Could you check a few things on this model? Use its own coordinates, in mm. Give positions to 0.01 mm unless a question says otherwise; leave off trailing zeros. Order: outer loops, then holes, each group sorted by start corner. A loop starts at its lowest first (then second) coordinate and runs counter-clockwise, first axis right, second up. Notation, with made-up numbers: (30.5, 29) - (71.5, 29) arc R19 cw to (71.5, 50) - close; hole circle Ø5 at (23, 59.5). An arc over 180 degrees is marked (long way). One line per question, with ' | ' between items. Start each with the question number.
1. For P1, Ø2, axis at y = -21, z = 1.5, coming from the -X side; P2, Ø1.6, axis at x = -21, z = 1.5, coming from the -Y side; P3, Ø3, axis at x = 10, y = 0, coming from the -Z side; P4, Ø4, axis at y = -3, z = 6, coming from the +X side, each with a flat end and sliding along its axis, tell me the tip position at first contact or that it passes through.
2. If we mould it in two halves opening along X, with no side actions, what happens to faces 1 (the flat face through (-21, 0.75, 1)), 2 (the flat face through (0, -5, 10)), 3 (the cylindrical face through (-0.228, -8.265, 6.056))? For each: released by +X, released by -X, zero draft, split by the parting line, or undercut.
3. Imagine slicing it at C-C (z = 3.5). Please give me the cut outline in (x, y).
4. I need wall thicknesses on probe 1 along Y at (x, z) = (0, 6); probe 2 along Y at (x, z) = (19, 1.25); probe 3 along Z at (x, y) = (18.5, 3). Which ranges of each line are inside material? Lowest first, please. Write a range as from..to.
5. Imagine slicing it at A-A (y = 0). Please give me the cut outline in (x, z), and give its area (3 significant figures).
```python
from build123d import *

# Parameters (mm, degrees)
SKETCH1_R           = 25
BOSS_EXTRUDE1_DEPTH = 10
SKETCH2_R           = 23
CUT_EXTRUDE1_DEPTH  = 2
SKETCH3_R           = 4
SKETCH3_R_2         = 1.75
CUT_EXTRUDE2_DEPTH  = 37.742346142
BOSS_EXTRUDE2_START = 2
BOSS_EXTRUDE2_DEPTH = 2
CIRPATTERN1_COUNT   = 20


with BuildPart() as part:
    # Sketch1 → Boss-Extrude1 (new body)
    with BuildSketch(Plane.XY):
        Circle(SKETCH1_R)
    extrude(amount=BOSS_EXTRUDE1_DEPTH)

    # Sketch2 → Cut-Extrude1 (cut)
    with BuildSketch(Plane(origin=(0, 0, 0), x_dir=(-1, 0, 0), z_dir=(0, 0, -1))):
        Circle(SKETCH2_R)
    extrude(amount=-CUT_EXTRUDE1_DEPTH, mode=Mode.SUBTRACT)

    # Sketch3 → Cut-Extrude2 (cut, through all)
    with BuildSketch(Plane.XY.offset(10)):
        Circle(SKETCH3_R)
        with Locations((10, 0)):
            Circle(SKETCH3_R_2)
        with Locations((0, -10)):
            Circle(SKETCH3_R_2)
        with Locations((-10, 0)):
            Circle(SKETCH3_R_2)
        with Locations((0, 10)):
            Circle(SKETCH3_R_2)
    extrude(amount=-CUT_EXTRUDE2_DEPTH, mode=Mode.SUBTRACT)

    # Sketch4 → Boss-Extrude2 (add)
    with BuildSketch(Plane(origin=(0, 0, 2), x_dir=(-1, 0, 0), z_dir=(0, 0, -1)).offset(BOSS_EXTRUDE2_START)):
        with BuildLine():
            Line((-0.75, 22.987768487), (-0.75, 18.464528853))
            Line((-0.75, 18.464528853), (0.75, 18.464528853))
            Line((0.75, 18.464528853), (0.75, 22.987768487))
            ThreePointArc((0.75, 22.987768487), (0, 23), (-0.75, 22.987768487))
        make_face()
    boss_extrude2 = extrude(amount=-BOSS_EXTRUDE2_DEPTH)

    # CirPattern1: Boss-Extrude2 ×20 about axis
    cirpattern1_axis = Axis((0, 0, 0), (0, 0, 1))
    for i in range(1, CIRPATTERN1_COUNT):
        add(boss_extrude2.rotate(cirpattern1_axis, i * 360 / CIRPATTERN1_COUNT))


solid = part.part
```
Results found:
1) P1: stops at x = -15 | P2: stops at y = -14.73 | P3: passes through | P4: stops at x = 24.98
2) face 1: undercut | face 2: zero draft | face 3: undercut
3) outline: circle Ø50 at (0, 0); hole circle Ø3.5 at (-10, 0); hole circle Ø8 at (0, 0); hole circle Ø3.5 at (0, -10); hole circle Ø3.5 at (0, 10); hole circle Ø3.5 at (10, 0)
4) probe 1: y = -25..-11.75, -8.25..-4, 4..8.25, 11.75..25 | probe 2: y = -16.25..-12.88, -6.96..-5.38, -0.75..0.75, 5.38..6.96, 12.88..16.25 | probe 3: z = 2..10
5) outline: (-25, 0) - (-18.46, 0) - (-18.46, 2) - (-11.75, 2) - (-11.75, 10) - (-25, 10) - close; (-8.25, 2) - (-4, 2) - (-4, 10) - (-8.25, 10) - close; (4, 2) - (8.25, 2) - (8.25, 10) - (4, 10) - close; (11.75, 2) - (18.46, 2) - (18.46, 0) - (25, 0) - (25, 10) - (11.75, 10) - close | area: 306 mm2
